Could you check a few things on this drawing? It's one solid part, dimensions in mm from its lowest x, y, z. Give positions to 0.01 mm unless a question says otherwise; leave off trailing zeros. Write each loop counter-clockwise with the first axis right and the second up, starting at its lowest first coordinate (ties: lowest second). Pieces come first, ordered by that corner, then holes. Notation, with made-up numbers: (-21, -15) - (8, -15) arc R23 cw to (8, 12) - close; hole circle Ø7 at (30.25, -17.75). An arc over 180 degrees is marked (long way). One line per item, written item: value. Start each with the question number.
1) Imagine slicing it at D-D on x = 51. Write out the boundary of the cut face in (y, z).
2) Imagine slicing it at B-B on z = 0.7. Write out the boundary of the cut face in (x, y) (1 decimal), plus the area to 3 significant figures.
3) Imagine slicing it at C-C on y = 12. Write out the boundary of the cut face in (x, z) (1 decimal).
4) Please list where these lines run through material, in increasing order: L1, parallel to Y at x = 71.5, z = 0.75; L2, parallel to Y at x = 32, z = 0.6 (1 decimal); L3, parallel to Y at x = 16.5, z = 0.45 (1 decimal). Write a range as [from, to].
5) I'm going to push a flat-ended pin straight in: P1, Ø2.5, axis at x = 79.75, y = 17.5, coming from the +Z side. Where does the tip first touch, or does it pass through?
6) Imagine slicing it at A-A on x = 19. Write out the boundary of the cut face in (y, z), plus the area to 3 significant figures.
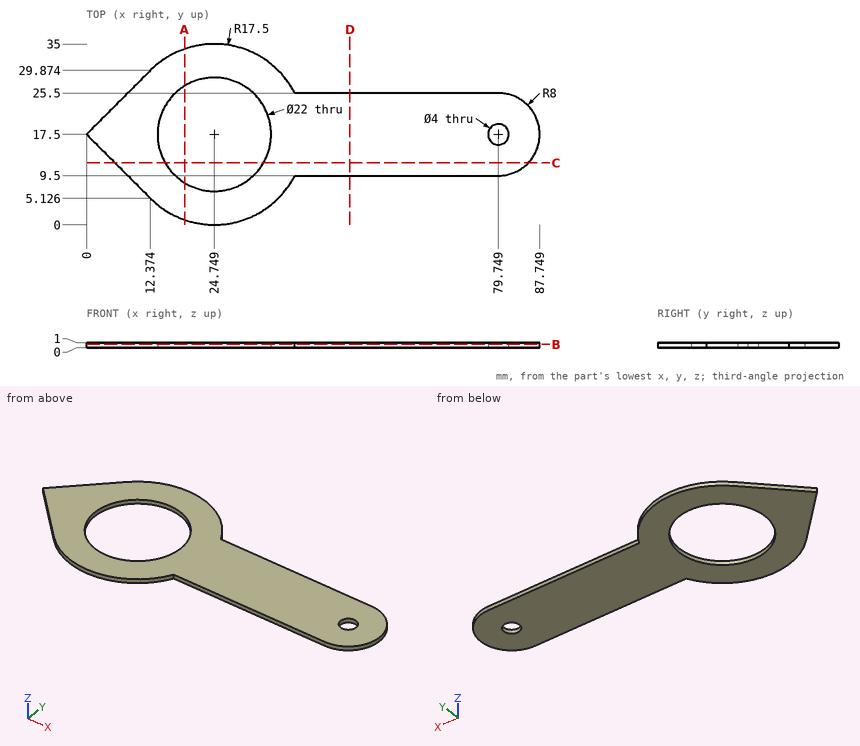
Numbers:
1. outline: (9.5, 0) - (25.5, 0) - (25.5, 1) - (9.5, 1) - close
2. outline: (0, 17.5) - (12.4, 5.1) arc R17.5 ccw to (40.3, 9.5) - (79.7, 9.5) arc R8 ccw to (87.7, 17.5) arc R8 ccw to (79.7, 25.5) - (40.3, 25.5) arc R17.5 ccw to (12.4, 29.9) - close; hole circle Ø22 at (24.7, 17.5); hole circle Ø4 at (79.7, 17.5)
2. area: 1,350 mm^2
3. outline: (5.5, 0) - (15.2, 0) - (15.2, 1) - (5.5, 1) - close; (34.3, 0) - (85.6, 0) - (85.6, 1) - (34.3, 1) - close
4. L1: [9.5, 25.5]
4. L2: [1.6, 9.2], [25.8, 33.4]
4. L3: [2.1, 10.2], [24.8, 32.9]
5. P1: through
6. outline: (0.97, 0) - (8.12, 0) - (8.12, 1) - (0.97, 1) - close; (26.88, 0) - (34.03, 0) - (34.03, 1) - (26.88, 1) - close
6. area: 14.3 mm^2
